Design review of the part built by this model. Coordinates are the model's own, in mm. Give positions to 0.01 mm unless a question says otherwise; leave off trailing zeros. Write each loop counter-clockwise with the first axis right and the second up, starting at its lowest first coordinate (ties: lowest second). Pieces come first, ordered by that corner, then holes. Notation, with made-up numbers: M 66.5,7.25 L 113.5,7.25 A12 cw 113.5,15.25 Z; hole C 79,65 d8. An arc over 180 degrees is marked long. Answer in a Markdown table with one row per item.
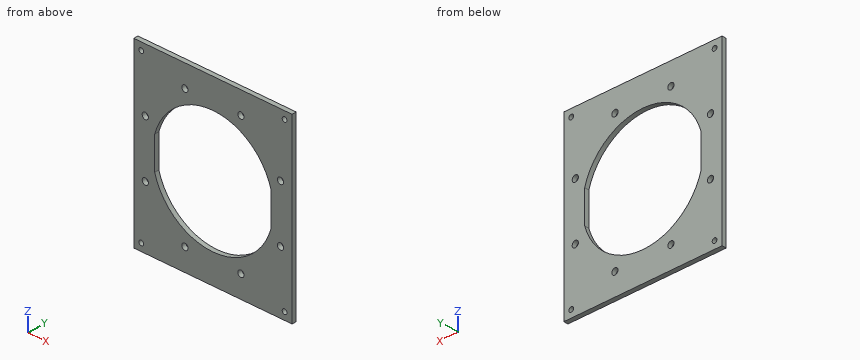
Autodesk Inventor part; units mm, degrees
ref_plane "YZ Plane" through (0, 0, 0) normal (1, 0, 0) x (0, 1, 0)
ref_plane "XZ Plane" through (0, 0, 0) normal (0, 1, 0) x (-1, 0, 0)
ref_plane "XY Plane" through (0, 0, 0) normal (0, 0, 1) x (1, 0, 0)
sketch "スケッチ1" plane through (0, 0, 0) normal (0, 1, 0) x (-1, 0, 0)
  line L0 (0, 0) -> (106, 0)
  line L1 (106, 0) -> (106, -120)
  line L2 (106, -120) -> (0, -120)
  line L3 (0, -120) -> (0, 0)
  dimension "d0" = 106
  dimension "d1" = 120
extrude "押し出し1" add sketch "スケッチ1" along normal blind 3
sketch "スケッチ2" plane through (0, 3, 0) normal (0, 1, 0) x (1, 0, 0)
  line L0 (-106, 120) -> (-106, 0)
  line L1 (0, 120) -> (-106, 120)
  line L2 (-106, 0) -> (0, 120)
  circle A0 centre (-53, 60) radius 49
  line L3 (-106, 60) -> (0, 60)
  line L4 (0, 0) -> (0, 120)
  line L5 (-53, 60) -> (-7.7299, 78.7515)
  point P0 (-34.2485, 105.2701)
  point P1 (-71.7515, 105.2701)
  point P2 (-98.2701, 78.7515)
  point P3 (-98.2701, 41.2485)
  point P4 (-71.7515, 14.7299)
  point P5 (-34.2485, 14.7299)
  point P6 (-7.7299, 41.2485)
  dimension "d4" = 98
  dimension "d5" = 22.5
  dimension "d8" = 360
hole "穴1" at (-7.7299, 3, -78.7515) at (-34.2485, 3, -105.2701) at (-71.7515, 3, -105.2701) at (-98.2701, 3, -78.7515) at (-98.2701, 3, -41.2485) at (-71.7515, 3, -14.7299) at (-34.2485, 3, -14.7299) at (-7.7299, 3, -41.2485) direction (0, -1, 0) diameter 4.2 end through all
sketch "スケッチ3" plane through (0, 3, 0) normal (0, 1, 0) x (1, 0, 0)
  line L0 (-106, 120) -> (-106, 0)
  line L1 (0, 120) -> (-106, 120)
  line L2 (-106, 0) -> (0, 120)
  circle A0 centre (-53, 60) radius 40.5
  line L3 (-106, 0) -> (0, 0)
  line L4 (-92, 0) -> (-92, 120)
  line L5 (-14, 0) -> (-14, 120)
  point P0 (-14, 60)
  point P1 (-92, 70.9202)
  point P2 (-92, 49.0798)
  point P3 (-14, 49.0798)
  point P4 (-14, 70.9202)
  dimension "d17" = 81
  dimension "d20" = 39
  dimension "d21" = 39
extrude "押し出し2" cut sketch "スケッチ3" against normal blind 3 contours A0 L2 L4 | L2 A0 L5 picked at (-69.0671, 72.6536) picked at (-40, 56.3599)
sketch "スケッチ4" plane through (0, 3, 0) normal (0, 1, 0) x (1, 0, 0)
  line L0 (-106, 120) -> (-106, 0)
  line L1 (-106, 5) -> (0, 5)
  line L2 (0, 0) -> (0, 120)
  line L3 (-120, 115) -> (0, 115)
  line L4 (-106, 0) -> (0, 0)
  line L5 (0, 120) -> (-106, 120)
  line L6 (-106, 0) -> (0, 0)
  line L7 (-101, 0) -> (-101, 120)
  line L8 (-5, 120) -> (-5, 0)
  point P0 (-101, 5)
  point P1 (-5, 5)
  point P2 (-5, 115)
  point P3 (-101, 115)
  dimension "d22" = 5
  dimension "d23" = 5
  dimension "d24" = 5
  dimension "d25" = 5
hole "穴2" at (-101, 3, -5) at (-5, 3, -5) at (-5, 3, -115) at (-101, 3, -115) direction (0, -1, 0) diameter 3.2 end through all
equation "\"d15\" = Thickness"
equation "\"BendRadius\" = Thickness"
equation "\"BendReliefWidth\" = Thickness"
equation "\"BendReliefDepth\" = 0.5 * Thickness"
equation "\"CornerReliefSize\" = 4 * Thickness"
equation "\"MinimumRemnant\" = 2 * Thickness"
equation "\"TransitionRadius\" = BendRadius"
equation "\"JacobiRadiusSize\" = BendRadius"
equation "\"GapSize\" = Thickness"
properties part number "link2_plate2" material "アルミニウム 6061"
1) Add section C-C (x = -79.5). Write out the cut boundary in (y, z), and give its area (3 significant figures).
Geometry says:
| item | result |
|---|---|
| outline | M 0,-120 L 3,-120 L 3,-90.63 L 0,-90.63 Z; M 0,-29.37 L 3,-29.37 L 3,0 L 0,0 Z |
| area | 176 mm^2 |
2) Add section A-A (z = -60.5). Write out the cut boundary in (x, y), and give its area (3 significant figures).
Geometry says:
| item | result |
|---|---|
| outline | M -106,0 L -92,0 L -92,3 L -106,3 Z; M -14,0 L 0,0 L 0,3 L -14,3 Z |
| area | 84.0 mm^2 |
3) To check wall thickness, follow probe 1 along X at (y, z) = (2, -115); probe 2 along X at (y, z) = (0.85, -67); probe 3 along X at (y, z) = (1.1, -5.5). State the ranges of each line that lie inside material, in increasing order. Write a range as [from, to].
Geometry says:
| item | result |
|---|---|
| probe 1 | [-106, -102.6], [-99.4, -6.6], [-3.4, 0] |
| probe 2 | [-106, -92], [-14, 0] |
| probe 3 | [-106, -102.52], [-99.48, -6.52], [-3.48, 0] |
4) Add section D-D (y = 1.55). Count the separate pieces of the cut face and the enclosed holes in it, and give its area (3 significant figures).
Geometry says:
| item | result |
|---|---|
| separate pieces | 1 |
| enclosed holes | 13 |
| area | 7,470 mm^2 |
5) Add section B-B (z = -5). Write out the cut boundary in (x, y), and give its area (3 significant figures).
Geometry says:
| item | result |
|---|---|
| outline | M -106,0 L -102.6,0 L -102.6,3 L -106,3 Z; M -99.4,0 L -6.6,0 L -6.6,3 L -99.4,3 Z; M -3.4,0 L 0,0 L 0,3 L -3.4,3 Z |
| area | 299 mm^2 |
